Autodesk Inventor part; units mm, degrees
ref_plane "YZ Plane" through (0, 0, 0) normal (1, 0, 0) x (0, 1, 0)
ref_plane "XZ Plane" through (0, 0, 0) normal (0, 1, 0) x (-1, 0, 0)
ref_plane "XY Plane" through (0, 0, 0) normal (0, 0, 1) x (1, 0, 0)
sketch "Sketch1" plane through (0, 0, 0) normal (0, 1, 0) x (-1, 0, 0)
  circle A0 centre (0, 0) radius 0.36
  circle A1 centre (0, 0) radius 5
  dimension "d2" = 10
  dimension "d24" = 0.72
extrude "Extrusion1" add sketch "Sketch1" along normal blind 6.275
sketch "Sketch2" plane through (0, 6.275, 0) normal (0, 1, 0) x (1, 0, 0)
  circle A0 centre (0, 0) radius 2.5
  dimension "d10" = 5
sketch "Sketch3" plane through (0, 0, 0) normal (0, -1, 0) x (1, 0, 0)
  line L0 (-1.775, 1.775) -> (1.775, 1.775)
  line L1 (1.775, 1.775) -> (1.775, -1.775)
  line L2 (1.775, -1.775) -> (-1.775, -1.775)
  line L3 (-1.775, -1.775) -> (-1.775, 1.775)
  line L4 (-1.775, 1.775) -> (1.775, -1.775) construction
  line L5 (1.775, 1.775) -> (-1.775, -1.775) construction
  arc A0 (1.775, 1.475) -> (1.475, 1.775) centre (1.775, 1.775) ccw
  arc A1 (1.475, -1.775) -> (1.775, -1.475) centre (1.775, -1.775) ccw
  arc A2 (-1.775, -1.475) -> (-1.475, -1.775) centre (-1.775, -1.775) ccw
  arc A3 (-1.475, 1.775) -> (-1.775, 1.475) centre (-1.775, 1.775) ccw
  point P0 (0, 0)
  dimension "d11" = 0.3
  dimension "d12" = 3.55
extrude "Extrusion2" cut sketch "Sketch3" against normal blind 1.275
sketch "Sketch5" plane through (0, 0, 0) normal (0, 0, 1) x (1, 0, 0)
  line L0 (-0.36, 1.275) -> (0.36, 1.275)
  line L1 (5, 6.275) -> (-5, 6.275)
  arc A0 (-0.36, 1.275) -> (-2.5, 6.275) centre (-11.8917, -0.7026) ccw
  line L2 (0, 1.275) -> (0, 6.275)
  line L3 (0.36, 1.275) -> (0, 1.275)
  line L4 (0.36, 6.275) -> (0.36, 1.275)
  line L5 (0.36, 6.275) -> (-2.5, 6.275)
  point P0 (0, 0)
  dimension "d17" = 2.5
  dimension "d23" = 11.7
revolve "Revolution1" cut sketch "Sketch5" angle 360 about axis through (0, 1.275, 0) along (0, 1, 0) contours A0 L1 L2 L0
fillet "Fillet1" radius 0.05 1 edges at (0.36, 1.275, 0)
properties part number "Acoustic Horn 30deg V1"
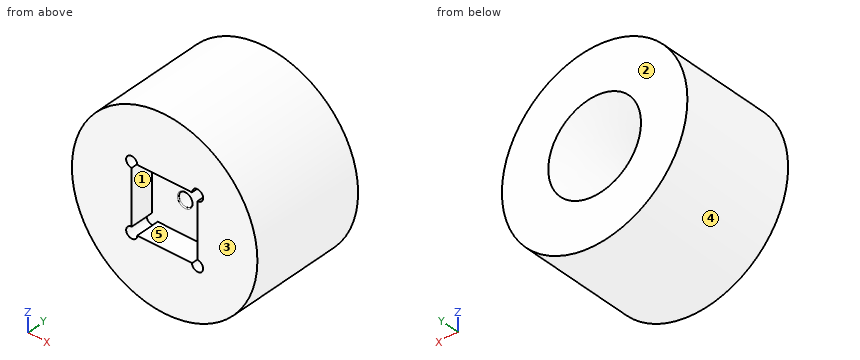
Build history of the part. All positions in model axes, mm. Face numbers are marked on the shaded views. A direction names the side the tool comes from. Give positions to 0.01 mm unless a question says otherwise; leave off trailing zeros. Order: outer loops, then holes, each group sorted by start corner. A loop starts at its lowest first (then second) coordinate and runs counter-clockwise, first axis right, second up. Notation, with made-up numbers: M 76,-10 L 109,-10 A8 ccw 109,-2 Z; hole C -39.5,29 d8. An arc over 180 degrees is marked long. Use one line per item in the form item = value.
1) Drop flat-ended pins along their axis: pin 1 (3 mm diameter, centred on x = -0.5, z = 3, fed in from -Y); pin 2 (3 mm diameter, centred on x = 3, y = 2.5, fed in from -Z); pin 3 (1.2 mm diameter, centred on x = -0.5, z = 1, fed in from -Y) (3 decimals). Give the stop position or say it passes through.
Calculated:
pin_1 = 0
pin_2 = -4.77
pin_3 = 1.275
2) Saw through at D-D (x = 3.5). Give the cut face in (y, z) (3 decimals), plus the area to 3 significant figures.
Calculated:
outline = M 0,-3.571 L 6.275,-3.571 L 6.275,3.571 L 0,3.571 Z
area = 44.8 mm2
3) Saw through at B-B (z = -2.75). Give the cut face in (x, y) (3 decimals), plus the area to 3 significant figures.
Calculated:
outline = M -4.176,0 L 4.176,0 L 4.176,6.275 L -4.176,6.275 Z
area = 52.4 mm2
4) Probe probe 1 along X at (y, z) = (4.5, -0.25); probe 2 along Z at (x, y) = (0.5, 2.25); probe 3 along Z at (x, y) = (0.75, 5). List the from-to ranges inside material, lowest first.
Calculated:
probe_1 = -4.99 to -1.39, 1.39 to 4.99
probe_2 = -4.97 to -0.27, 0.27 to 4.97
probe_3 = -4.94 to -1.5, 1.5 to 4.94
5) Two-plate mould, pull along Z, no slides. Class the marked faces 3, 4 and 5: released by +Z, released by -Z, zero draft, split by the parting line, or undercut.
Calculated:
face_3 = zero draft
face_4 = split by the parting line
face_5 = undercut
6) Tool access for the marked faces 1 and 2: list every direction of +Z, -Z, +X, -X, +Y, -Y with a clear straight run to the whole face (end or side of a thin tool).
Calculated:
face_1 = -Y
face_2 = +Z, -Z, +X, -X, +Y
7) Saw through at A-A (y = 0.5). Give the cut face in (x, z) (3 decimals).
Calculated:
outline = C 0,0 d10; hole M -1.775,-1.475 A0.3 ccw long -1.475,-1.775 L 1.475,-1.775 A0.3 ccw long 1.775,-1.475 L 1.775,1.475 A0.3 ccw long 1.475,1.775 L -1.475,1.775 A0.3 ccw long -1.775,1.475 Z
8) Saw through at C-C (y = 3.75). Give the cut face in (x, z).
Calculated:
outline = C 0,0 d10; hole C 0,0 d2.14
